The model under review builds one solid part; all positions refer to its coordinate system, in mm. A direction names the side the tool comes from. Coordinates: 2 decimals unless noted, no trailing zeros. Order: outer loops, then holes, each group sorted by start corner. A loop starts at its lowest first (then second) coordinate and runs counter-clockwise, first axis right, second up. Notation, with made-up numbers: M 60,14 L 81,14 A28 ccw 81,34 Z; hole C 18.25,37 d5. An arc over 180 degrees is marked long. Write each question's results on one line, items separated by ' | '.
from build123d import *

# Parameters (mm, degrees)
SKETCH1_W                      = 100
SKETCH1_H                      = 32
SKETCH1_R                      = 3.96875
BOSS_EXTRUDE1_DEPTH            = 10
FILLET1_R                      = 15
CBORE_FOR_M3_SHCS_D            = 3.4
CBORE_FOR_M3_SHCS_DEPTH        = 23
CBORE_FOR_M3_SHCS_CBORE_D      = 6.5
CBORE_FOR_M3_SHCS_CBORE_DEPTH  = 3
CBORE_FOR_M3_SHCS_TIP          = 1.021463052
CBORE_FOR_M3_SHCS1_D           = 3.4
CBORE_FOR_M3_SHCS1_DEPTH       = 23
CBORE_FOR_M3_SHCS1_CBORE_D     = 6.5
CBORE_FOR_M3_SHCS1_CBORE_DEPTH = 3
CBORE_FOR_M3_SHCS1_TIP         = 1.021463052


with BuildPart() as part:
    # Sketch1 → Boss-Extrude1 (new body)
    with BuildSketch(Plane(origin=(0, 0, 0), x_dir=(0, 0, -1), z_dir=(1, 0, 0))):
        Rectangle(SKETCH1_W, SKETCH1_H)
        with Locations((-30, 4)):
            Circle(SKETCH1_R, mode=Mode.SUBTRACT)
    extrude(amount=BOSS_EXTRUDE1_DEPTH)

    # Fillet1
    fillet1_edges = [part.edges().sort_by_distance(p)[0] for p in [
        (5, -16, 50),
    ]]
    fillet(fillet1_edges, radius=FILLET1_R)

    # CBORE for M3 SHCS
    with Locations(Plane(origin=(-616.293536786, 26, -1323.282701689), x_dir=(1, 0, 0), z_dir=(0, 1, 0))):
        with Locations((731.293536786, -1281.282701689), (731.293536786, -1343.282701689), (621.293536786, -1281.282701689), (621.293536786, -1365.282701689), (621.293536786, -1323.282701689), (731.293536786, -1312.282701689)):
            CounterBoreHole(CBORE_FOR_M3_SHCS_D / 2, CBORE_FOR_M3_SHCS_CBORE_D / 2, CBORE_FOR_M3_SHCS_CBORE_DEPTH, depth=CBORE_FOR_M3_SHCS_DEPTH)
            with Locations((0, 0, -(CBORE_FOR_M3_SHCS_DEPTH + CBORE_FOR_M3_SHCS_TIP / 2))):  # 118° drill point
                Cone(0, CBORE_FOR_M3_SHCS_D / 2, CBORE_FOR_M3_SHCS_TIP, mode=Mode.SUBTRACT)

    # CBORE for M3 SHCS1
    with Locations(Plane(origin=(0, -904.012147263, -1323.282701689), x_dir=(0, 0, 1), z_dir=(-1, 0, 0))):
        with Locations((1281.282701689, 893.012147263), (1325.282701689, 893.012147263), (1303.282701689, 893.012147263)):
            CounterBoreHole(CBORE_FOR_M3_SHCS1_D / 2, CBORE_FOR_M3_SHCS1_CBORE_D / 2, CBORE_FOR_M3_SHCS1_CBORE_DEPTH, depth=CBORE_FOR_M3_SHCS1_DEPTH)
            with Locations((0, 0, -(CBORE_FOR_M3_SHCS1_DEPTH + CBORE_FOR_M3_SHCS1_TIP / 2))):  # 118° drill point
                Cone(0, CBORE_FOR_M3_SHCS1_D / 2, CBORE_FOR_M3_SHCS1_TIP, mode=Mode.SUBTRACT)


solid = part.part
1) To check wall thickness, follow line 1 along Z through (x, y) = (5, 8); line 2 along Y through (x, z) = (4.5, 2); line 3 along X through (y, z) = (11.75, 42). State the ranges of each line that lie inside material, in increasing order.
Solutions:
line 1: -50 to -43.7, -40.3 to -1.7, 1.7 to 40.3, 43.7 to 50 | line 2: -16 to -12.7, -9.3 to 16 | line 3: 0 to 3.3, 6.7 to 10
2) For faces 1 (the cylindrical face through (6.55, -12.03, -40.65)), 2 (the flat face through (3, -12.4, -40.6)), 3 (the cylindrical face through (5.37, 9.41, -40.34)), list the 3-axis set-ups (+Z, -Z, +X, -X, +Y, -Y) from which the entire face can be reached by the end or side of a thin tool; tool diameter is ignored.
Solutions:
face 1: +X, -X | face 2: -X | face 3: +Y
3) Take a section at B-B on x = 8.5. State the section outline as (y, z) points.
Solutions:
outline: M -16,-50 L 16,-50 L 16,50 L -1,50 A15 ccw -16,35 Z; hole C -11,-42 d3.4; hole C -11,-20 d3.4; hole C -11,2 d3.4; hole C 4,30 d7.94
4) Take a section at C-C on z = 32.5. State the section outline as (x, y) points.
Solutions:
outline: M 0,-16 L 10,-16 L 10,0.92 L 0,0.92 Z; M 0,7.08 L 10,7.08 L 10,16 L 0,16 Z
5) For pin 1 (4.5 mm diameter, centred on y = -11, z = -42, fed in from -X); pin 2 (4 mm diameter, centred on y = -11, z = 2, fed in from +X); pin 3 (5.5 mm diameter, centred on x = 5, z = 42, fed in from -Y); pin 4 (2.5 mm diameter, centred on x = 5, z = 0, fed in from +Y), all flat-tipped, find the tip position at first contact; note any pin that passes through.
Solutions:
pin 1: x = 3 | pin 2: x = 10 | pin 3: y = -15.39 | pin 4: y = 2.73
6) The part is to be moulded in two halves that separate along Y. For faces 4 (the conical face through (4.962, 2.156, -42.293)), 5 (the cylindrical face through (1.479, -7.778, 1.577)), 6 (the flat face through (0, 0, 1)), say which applies: pulls with the +Y half, pulls with the -Y half, needs draft (parallel to the pull), parting line crosses it, or undercut.
Solutions:
face 4: pulls with the +Y half | face 5: undercut | face 6: needs draft
7) Take a section at A-A on y = 4. State the section outline as (x, z) points.
Solutions:
outline: M 0,-50 L 10,-50 L 10,26.03 L 0,26.03 Z; M 0,33.97 L 10,33.97 L 10,50 L 0,50 Z; hole C 5,-42 d3.4; hole C 5,0 d3.4; hole C 5,42 d3.4
